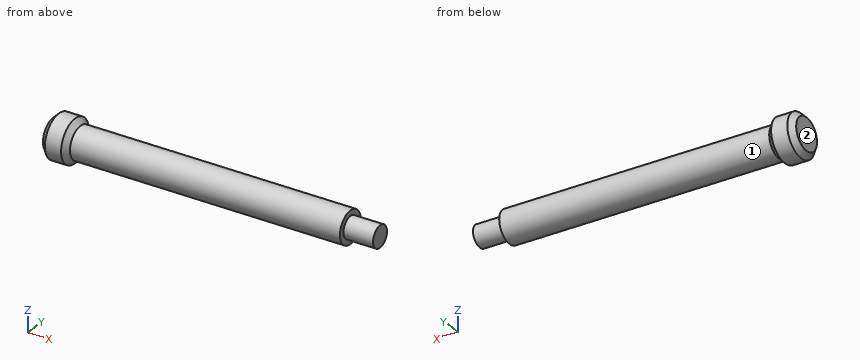
Autodesk Inventor part; units mm, degrees
ref_plane "YZ Plane" through (0, 0, 0) normal (1, 0, 0) x (0, 1, 0)
ref_plane "XZ Plane" through (0, 0, 0) normal (0, 1, 0) x (-1, 0, 0)
ref_plane "XY Plane" through (0, 0, 0) normal (0, 0, 1) x (1, 0, 0)
sketch "Sketch1" plane through (0, 0, 0) normal (0, 0, 1) x (1, 0, 0)
  line L0 (0, 0) -> (60.5, 0)
  line L1 (60.5, 0) -> (60.5, 3)
  line L2 (60.5, 3) -> (0, 3)
  line L3 (0, 3) -> (0, 0)
  line L4 (60.5, 0) -> (55, 0)
  line L5 (55, 0) -> (55, 2)
  line L6 (55, 2) -> (60.5, 2)
  line L7 (60.5, 2) -> (60.5, 0)
  line L8 (55, 2) -> (55, 3)
  line L9 (0, 0) -> (5, 0)
  line L10 (5, 0) -> (5, 4)
  line L11 (5, 4) -> (0, 4)
  line L12 (0, 4) -> (0, 0)
  point P0 (5, 3)
  dimension "d0" = 60.5
  dimension "d1" = 3
  dimension "d2" = 5.5
  dimension "d3" = 2
  dimension "d4" = 5
  dimension "d5" = 4
revolve "Revolution1" add sketch "Sketch1" angle 360 about axis through (0, 0, 0) along (1, 0, 0) contours L3 L2 L10 L0 | L10 L2 L8 L5 L0 | L12 L11 L10 L2 | L5 L6 L1 L0
chamfer "Chamfer1" distance 1 angle 45 2 edges at (5, -4, 0) (0, -4, 0)
properties part number "Hajtókar1"
Check sheet for the modelled part. Datum: model origin and axes. Units: mm. Face numbers are marked on the shaded views. A direction names the side the tool comes from. Coordinates: 2 decimals unless noted, no trailing zeros. Write each loop counter-clockwise with the first axis right and the second up, starting at its lowest first coordinate (ties: lowest second). Pieces come first, ordered by that corner, then holes. Notation, with made-up numbers: M 22,-5 L 41,-5 A22 cw 41,32 Z; hole C 7.25,-31.5 d6. An arc over 180 degrees is marked long. Use one line per item in the form item = value.
Item 1: Sectioned sample at C-C, the plane x = 16.5. Record the cut outline in (y, z).
Answer below:
outline = C 0,0 d6
Item 2: Set-up check for the marked faces 1 and 2: record each of +Z, -Z, +X, -X, +Y, -Y from which the full face is reachable in a straight line by a thin tool's end or side.
Answer below:
face_1 = +X
face_2 = +Z, -Z, -X, +Y, -Y
Item 3: Sectioned sample at D-D, the plane x = 55.5. Record the cut outline in (y, z).
Answer below:
outline = C 0,0 d4
Item 4: Gauge pin test, flat ends, axial feed: pin 1 Ø2 at (x, y) = (19.5, -1) entering from +Z; pin 2 Ø2 at (x, y) = (51.5, -3) entering from +Z; pin 3 Ø1.5 at (x, z) = (19.5, -2.5) entering from -Y. Record the tip position at first contact, or that the pin passes through.
Answer below:
pin_1 = 3
pin_2 = 2.24
pin_3 = -2.44
Item 5: Material ranges on L1, parallel to Z at x = 49, y = -0.25; L2, parallel to X at y = 1, z = -2.5; L3, parallel to Y at x = 50.5, z = -2, recorded low to high. Write a range as from..to.
Answer below:
L1 = -2.99..2.99
L2 = 0..55
L3 = -2.24..2.24
